Autodesk Inventor part; units mm, degrees
ref_plane "Work Plane1" through (-50.8, 1219.2, 482.6) normal (0, -1, 0) x (1, 0, 0)
ref_plane "Work Plane2" through (0, 0, 304.8) normal (0, 0, 1) x (1, 0, 0)
ref_plane "YZ Plane" through (0, 0, 0) normal (1, 0, 0) x (0, 1, 0)
sketch "Sketch1" plane through (0, 0, 0) normal (0, 0, 1) x (1, 0, 0)
  line L0 (0, 0) -> (127, 0)
  line L1 (127, 0) -> (127, 2438.4)
  line L2 (127, 2438.4) -> (0, 2438.4)
  line L3 (0, 2438.4) -> (0, 0)
  dimension "d0" = 127
  dimension "d1" = 2438.4
extrude "Extrusion1" add sketch "Sketch1" along normal blind 609.6
sketch "Sketch3" plane through (0, 0, 0) normal (-1, 0, 0) x (0, 0, 1)
  line L0 (609.6, 2438.4) -> (609.6, 0)
  line L1 (0, 2438.4) -> (0, 0)
  line L2 (0, 0) -> (609.6, 0)
  line L3 (609.6, 0) -> (609.6, 2438.4)
  line L4 (0, 0) -> (609.6, 0)
  line L5 (609.6, 0) -> (609.6, 812.8)
  line L6 (609.6, 812.8) -> (0, 812.8)
  line L7 (0, 812.8) -> (0, 0)
  dimension "d8" = 812.8
extrude "Extrusion3" add sketch "Sketch3" along normal blind 50.8
sketch "Sketch4" plane through (0, 2438.4, 0) normal (-1, 0, 0) x (0, 0, 1)
  line L0 (609.6, -1625.6) -> (0, -1625.6)
  line L1 (609.6, 0) -> (609.6, -1625.6)
  line L2 (0, 0) -> (0, -1625.6)
  line L3 (0, -1625.6) -> (609.6, -1625.6)
  line L4 (609.6, -1625.6) -> (609.6, -812.8)
  line L5 (609.6, -812.8) -> (0, -812.8)
  line L6 (0, -812.8) -> (0, -1625.6)
  point P0 (0, -2438.4)
  dimension "d11" = 812.8
extrude "Extrusion4" add sketch "Sketch4" along normal blind 127
sketch "Sketch5" plane through (0, 1625.6, 0) normal (-1, 0, 0) x (0, 0, 1)
  line L0 (519.5823, 575.5562) -> (519.5823, 226.8611) construction
  line L1 (519.5823, 226.8611) -> (23.9628, 226.8611) construction
  line L2 (23.9628, 226.8611) -> (23.9628, 575.5562) construction
  line L3 (23.9628, 575.5562) -> (519.5823, 575.5562) construction
  point P0 (0, -1625.6)
sketch "Sketch6" plane through (-127, 2438.4, 0) normal (-1, 0, 0) x (0, 0, 1)
  line L0 (504.953, -1049.3947) -> (504.953, -1386.624) construction
  line L1 (504.953, -1386.624) -> (88.8121, -1386.624) construction
  line L2 (88.8121, -1386.624) -> (88.8121, -1049.3947) construction
  line L3 (88.8121, -1049.3947) -> (504.953, -1049.3947) construction
  point P0 (0, -2438.4)
sketch "Sketch7" plane through (-50.8, 0, 0) normal (-1, 0, 0) x (0, 0, 1)
  line L0 (510.0659, 619.5124) -> (510.0659, 275.8757) construction
  line L1 (510.0659, 275.8757) -> (79.0869, 275.8757) construction
  line L2 (79.0869, 275.8757) -> (79.0869, 619.5124) construction
  line L3 (79.0869, 619.5124) -> (510.0659, 619.5124) construction
  point P0 (0, 0)
sketch "Sketch8" plane through (-50.8, 0, 0) normal (-1, 0, 0) x (0, 0, 1)
  line L0 (0, 812.8) -> (609.6, 812.8)
  line L1 (0, 0) -> (609.6, 0)
  line L2 (355.6, 812.8) -> (254, 812.8)
  line L3 (254, 812.8) -> (254, 0)
  line L4 (254, 0) -> (355.6, 0)
  line L5 (355.6, 0) -> (355.6, 812.8)
  line L6 (609.6, 0) -> (609.6, 812.8)
  line L7 (0, 812.8) -> (0, 0)
  point P0 (127, 0)
  point P1 (482.6, 0)
  point P2 (609.6, 127)
  point P3 (0, 127)
  dimension "d15" = 254
  dimension "d16" = 254
extrude "Extrusion5" add sketch "Sketch8" along normal up to surface (76.2 mm away) contours L0 L5 L1 L3
sketch "Sketch9" plane through (-127, 2438.4, 0) normal (-1, 0, 0) x (0, 0, 1)
  line L0 (254, -2438.4) -> (254, -1625.6)
  line L1 (355.6, -1625.6) -> (355.6, -2438.4)
  line L2 (609.6, -812.8) -> (0, -812.8)
  line L3 (355.6, -1625.6) -> (254, -1625.6)
  line L4 (254, -1625.6) -> (254, -812.8)
  line L5 (254, -812.8) -> (355.6, -812.8)
  line L6 (355.6, -812.8) -> (355.6, -1625.6)
  point P0 (0, -2438.4)
extrude "Extrusion6" add sketch "Sketch9" along normal blind 127
sketch "Sketch10" plane through (0, 1625.6, 0) normal (-1, 0, 0) x (0, 0, 1)
  line L0 (254, 0) -> (254, -812.8)
  line L1 (355.6, -812.8) -> (355.6, 0)
  line L2 (355.6, 0) -> (254, 0)
  line L3 (0, 812.8) -> (609.6, 812.8)
  line L4 (355.6, 0) -> (254, 0)
  line L5 (254, 0) -> (254, 812.8)
  line L6 (254, 812.8) -> (355.6, 812.8)
  line L7 (355.6, 812.8) -> (355.6, 0)
  point P0 (0, -1625.6)
  point P1 (127, 812.8)
  point P2 (482.6, 812.8)
extrude "Extrusion7" add sketch "Sketch10" along normal up to surface (254 mm away)
sketch "Sketch11" plane through (-127, 2438.4, 0) normal (-1, 0, 0) x (0, 0, 1)
  line L0 (254, -1625.6) -> (355.6, -1625.6)
  line L1 (254, -2438.4) -> (254, -1625.6)
  line L2 (355.6, -1625.6) -> (355.6, -2438.4)
  line L3 (355.6, -2438.4) -> (254, -2438.4)
  point P0 (0, -2438.4)
extrude "Extrusion8" add sketch "Sketch11" along normal up to surface (127 mm away)
ref_plane "Work Plane1" through (-50.8, 1219.2, 482.6) normal (0, -1, 0) x (1, 0, 0)
ref_plane "Work Plane2" through (0, 0, 304.8) normal (0, 0, 1) x (1, 0, 0)
sketch "Sketch15" plane through (-254, 2438.4, 0) normal (-1, 0, 0) x (0, 0, 1)
  line L0 (-285.5024, -2708.2595) -> (304.8, -2708.2595)
  line L1 (304.8, -2708.2595) -> (304.8, 202.5179)
  line L2 (304.8, 202.5179) -> (-285.5024, 202.5179)
  line L3 (-285.5024, 202.5179) -> (-285.5024, -2708.2595)
  line L4 (254, -2438.4) -> (254, 0)
  line L5 (355.6, 0) -> (355.6, -2438.4)
  point P0 (0, -2438.4)
  dimension "d55" = 50.8
  dimension "d56" = 50.8
extrude "Extrusion12" cut sketch "Sketch15" against normal blind 865.1875
equation "\"d8\" = 0.333333 * d1"
equation "\"d11\" = 0.333333 * d1"
properties part number "Hill"
Input: part model. Units: mm. Frame: model coordinates. A direction names the side the tool comes from. Coordinates: 2 decimals unless noted, no trailing zeros. Loops run counter-clockwise (first coordinate to the right, second up) from the corner with the lowest first, then second, coordinate; pieces in that order, holes last. Notation, with made-up numbers: (-31.5, -6.75) -> (20.5, -6.75) arc R28 ccw to (20.5, 15.25) -> close; hole circle Ø11 at (68.5, 13.5). An arc over 180 degrees is marked (long way). Use a Markdown table: item, result.
1) Cut plane C-C (x = -78). Return the cut outline in (y, z), then the cut area to 3 significant figures.
Results found:
| item | result |
|---|---|
| outline | (0, 304.8) -> (2438.4, 304.8) -> (2438.4, 355.6) -> (1625.6, 355.6) -> (1625.6, 609.6) -> (812.8, 609.6) -> (812.8, 355.6) -> (0, 355.6) -> close |
| area | 330,000 mm2 |
2) Access query for faces 1 (the flat face through (-254, 1236, 330)), 2 (the flat face through (-127, 1225, 481)), 3 (the flat face through (-63, 1625.6, 484)), 4 (the flat face through (-88, 812.8, 484)), 5 (the flat face through (24, 2438.4, 421)). Directions: +Z, -Z, +X, -X, +Y, -Y. A direction counts if a zero-diameter tool reaches every point of the face in a straight line with its end or side. Return the directions, or none.
Results found:
| item | result |
|---|---|
| face 1 | +Z, -Z, -X, +Y, -Y |
| face 2 | +Z, -X, +Y, -Y |
| face 3 | +Z, -X, +Y |
| face 4 | +Z, -X, -Y |
| face 5 | +Z, -Z, +X, -X, +Y |
3) Cut plane A-A (z = 479). Return the cut outline in (x, y).
Results found:
| item | result |
|---|---|
| outline | (-127, 812.8) -> (-50.8, 812.8) -> (-50.8, 0) -> (127, 0) -> (127, 2438.4) -> (0, 2438.4) -> (0, 1625.6) -> (-127, 1625.6) -> close |
4) Material intervals for line 1 along X through (y, z) = (1796, 549); line 2 along X through (y, z) = (991.5, 554); line 3 along Z through (x, y) = (-92, 768.5), sorted ascending. Write a range as from..to.
Results found:
| item | result |
|---|---|
| line 1 | x = 0..127 |
| line 2 | x = -127..127 |
| line 3 | z = 304.8..355.6 |
5) Contact query for flat-ended pins moving along their axis: pin 1 (6 mm diameter, centred on y = 570.5, z = 432, fed in from -X); pin 2 (1 mm diameter, centred on y = 1753.5, z = 380.5, fed in from -X); pin 3 (10 mm diameter, centred on x = -88.5, z = 490.5, fed in from +Y). Output: stop coordinate, or through.
Results found:
| item | result |
|---|---|
| pin 1 | stops at x = -50.8 |
| pin 2 | stops at x = 0 |
| pin 3 | stops at y = 1625.6 |
6) Cut plane B-B (y = 2052). Return the cut outline in (x, z), then the cut area to 3 significant figures.
Results found:
| item | result |
|---|---|
| outline | (-254, 304.8) -> (127, 304.8) -> (127, 609.6) -> (0, 609.6) -> (0, 355.6) -> (-254, 355.6) -> close |
| area | 51,600 mm2 |
7) Cut plane D-D (y = 1511). Return the cut outline in (x, z), then the cut area to 3 significant figures.
Results found:
| item | result |
|---|---|
| outline | (-254, 304.8) -> (127, 304.8) -> (127, 609.6) -> (-127, 609.6) -> (-127, 355.6) -> (-254, 355.6) -> close |
| area | 83,900 mm2 |
